Verification items for the finished model (mm, model axes). Give positions to 0.01 mm unless a question says otherwise; leave off trailing zeros. Order: outer loops, then holes, each group sorted by start corner. A loop starts at its lowest first (then second) coordinate and runs counter-clockwise, first axis right, second up. Notation, with made-up numbers: M 88,-3 L 115,-3 A9 cw 115,6 Z; hole C -8,-1.75 d4. An arc over 180 degrees is marked long. Answer as a JSON object with one key per item and string values.
```python
from build123d import *

# Parameters (mm, degrees)
SKETCH1_R           = 8
SKETCH1_R_2         = 3.175
SKETCH1_R_3         = 1.85
SKETCH1_R_4         = 4
BOSS_EXTRUDE1_DEPTH = 3.175
FILLET1_R           = 8
FILLET2_R           = 8


with BuildPart() as part:
    # Sketch1 → Boss-Extrude1 (new body)
    with BuildSketch(Plane.XY):
        with BuildLine():
            Line((176.640929786, -127.55), (67.815929786, -127.55))
            Line((67.815929786, -127.55), (67.815929786, -101.2))
            ThreePointArc((67.815929786, -101.2), (37.73889258, -51.561305416), (-20.184070214, -55.243498828))
            Line((-20.184070214, -55.243498828), (-20.184070214, -35.2))
            Line((-20.184070214, -35.2), (-23.359070214, -35.2))
            Line((-23.359070214, -35.2), (-23.359070214, 24.85))
            Line((-23.359070214, 24.85), (176.640929786, 24.85))
            Line((176.640929786, 24.85), (176.640929786, -127.55))
        make_face()
        with Locations((112.2, -41.275)):
            Circle(SKETCH1_R, mode=Mode.SUBTRACT)
        Circle(SKETCH1_R, mode=Mode.SUBTRACT)
        with Locations((11.43, -27.96)):
            Circle(SKETCH1_R_2, mode=Mode.SUBTRACT)
        with Locations((-11.43, 18.5)):
            Circle(SKETCH1_R_2, mode=Mode.SUBTRACT)
        with Locations((11.43, 18.5)):
            Circle(SKETCH1_R_2, mode=Mode.SUBTRACT)
        with Locations((45, -40)):
            Circle(SKETCH1_R_2, mode=Mode.SUBTRACT)
        with Locations((63.404393546, -6.8)):
            Circle(SKETCH1_R_2, mode=Mode.SUBTRACT)
        with Locations((108.95, -124.375)):
            Circle(SKETCH1_R_3, mode=Mode.SUBTRACT)
        with Locations((76.95, -124.375)):
            Circle(SKETCH1_R_3, mode=Mode.SUBTRACT)
        with Locations((-13.834070214, -43.2)):
            Circle(SKETCH1_R_2, mode=Mode.SUBTRACT)
        with Locations((84.102828318, 12.5)):
            Circle(SKETCH1_R_4, mode=Mode.SUBTRACT)
    extrude(amount=-BOSS_EXTRUDE1_DEPTH)

    # Fillet1
    fillet1_edges = [part.edges().sort_by_distance(p)[0] for p in [
        (67.815929786, -127.55, -1.5875),
    ]]
    fillet(fillet1_edges, radius=FILLET1_R)

    # Fillet2
    fillet2_edges = [part.edges().sort_by_distance(p)[0] for p in [
        (-23.359070214, 24.85, -1.5875),
    ]]
    fillet(fillet2_edges, radius=FILLET2_R)


solid = part.part
```
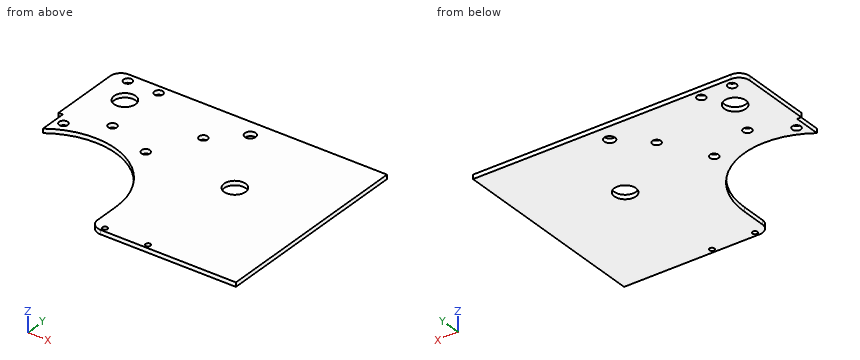
Q1. Section check D-D on y = -109.5. Record the cut outline in (x, z) (3 decimals), then the cut area to 3 significant figures.
Resolved:
{"outline": "M 67.816,-3.175 L 176.641,-3.175 L 176.641,0 L 67.816,0 Z", "area": "346 mm²"}
Q2. Section check B-B on z = -2.1. Count the separate pieces of the cut face and the enclosed holes in it, then the cut area to 3 significant figures.
Resolved:
{"separate pieces": "1", "enclosed holes": "11", "area": "23,000 mm²"}
Q3. Material ranges on L1, parallel to Y at x = -12, z = -1; L2, parallel to X at y = -40.5, z = -0.45; L3, parallel to Y at x = 112.2, z = -1.4 (3 decimals), recorded low to high.
Resolved:
{"L1": "y = -50.52 to -45.79, -40.61 to 15.38, 21.62 to 24.85", "L2": "x = -20.18 to -15.5, -12.16 to 41.86, 48.14 to 104.24, 120.16 to 176.64", "L3": "y = -127.55 to -49.275, -33.275 to 24.85"}
Q4. Gauge pin test, flat ends, axial feed: pin 1 Ø6.5 at (x, y) = (84.1, 12.5) entering from +Z; pin 2 Ø1.6 at (x, z) = (-21.5, -2) entering from -Y; pin 3 Ø1 at (y, z) = (-107.5, -2) entering from -X. Record the tip position at first contact, or that the pin passes through.
Resolved:
{"pin 1": "passes through", "pin 2": "stops at y = -35.2", "pin 3": "stops at x = 67.82"}
Q5. Section check A-A on y = -27.96. Record the cut outline in (x, z) (3 decimals), then the cut area to 3 significant figures.
Resolved:
{"outline": "M -23.359,-3.175 L 8.255,-3.175 L 8.255,0 L -23.359,0 Z; M 14.605,-3.175 L 176.641,-3.175 L 176.641,0 L 14.605,0 Z", "area": "615 mm²"}
Q6. Section check C-C on x = 0. Record the cut outline in (y, z) (3 decimals).
Resolved:
{"outline": "M -46.461,-3.175 L -8,-3.175 L -8,0 L -46.461,0 Z; M 8,-3.175 L 24.85,-3.175 L 24.85,0 L 8,0 Z"}
